Could you check a few things on this model? Use its own coordinates, in mm. A direction names the side the tool comes from. Round coordinates to 2 decimals unless told otherwise and drop trailing zeros. Write each loop counter-clockwise with the first axis right and the second up, starting at its lowest first coordinate (ties: lowest second). Pieces come first, ordered by that corner, then holes. Notation, with made-up numbers: (17.5, -0.5) - (43.5, -0.5) arc R15 ccw to (43.5, 14.5) - close; hole circle Ø11 at (34.25, 26). An arc over 180 degrees is marked (long way). Put each result on its own line as item: value.
Autodesk Fusion 360 part; units mm, degrees
sketch "Esquisse1" plane through (0, 0, 0) normal (0, 0, 1) x (1, 0, 0)
  line L0 (15.7988, 249.7948) -> (43.7076, 249.7948) construction
  line L1 (15.7988, 262.2639) -> (10.7166, 262.2639)
  line L2 (10.7166, 262.2639) -> (10.7166, 237.5139)
  line L3 (10.7166, 237.5139) -> (15.7988, 237.4198)
  line L4 (15.7988, 274.8948) -> (15.7988, 262.2639)
  line L5 (15.7988, 237.4198) -> (15.7988, 224.6948)
  line L6 (110.3988, 274.8948) -> (110.3988, 280.2948)
  line L7 (110.3988, 280.2948) -> (60.5988, 280.2948)
  line L8 (60.5988, 280.2948) -> (60.5988, 274.8948)
  line L9 (15.7988, 274.8948) -> (60.5988, 274.8948)
  line L10 (110.3988, 274.8948) -> (155.1988, 274.8948)
  line L11 (110.3988, 224.6948) -> (110.3988, 219.2948)
  line L12 (110.3988, 219.2948) -> (60.5988, 219.2948)
  line L13 (60.5988, 219.2948) -> (60.5988, 224.6948)
  line L14 (155.1988, 224.6948) -> (110.3988, 224.6948)
  line L15 (60.5988, 224.6948) -> (15.7988, 224.6948)
  line L16 (85.4988, 283.8421) -> (85.4988, 207.6137) construction
  line L17 (155.1988, 262.2639) -> (160.281, 262.2639)
  line L18 (160.281, 262.2639) -> (160.281, 237.5139)
  line L19 (160.281, 237.5139) -> (155.1988, 237.4198)
  line L20 (155.1988, 274.8948) -> (155.1988, 262.2639)
  line L21 (155.1988, 237.4198) -> (155.1988, 224.6948)
  circle A0 centre (13.4166, 249.7948) radius 1.6
  circle A1 centre (157.581, 249.7948) radius 1.6
  line L22 (33.7988, 274.8948) -> (37.1988, 274.8948)
  line L23 (37.1988, 274.8948) -> (37.1988, 268.8948)
  line L24 (33.7988, 268.8948) -> (33.7988, 274.8948)
  line L25 (35.4988, 277) -> (35.4988, 258) construction
  line L26 (32.7988, 268.8948) -> (32.7988, 266.1948)
  line L27 (38.1988, 266.1948) -> (38.1988, 268.8948)
  line L28 (37.1988, 266.1948) -> (37.1988, 264.6948)
  line L29 (36.6988, 264.1948) -> (34.2988, 264.1948)
  line L30 (33.7988, 264.6948) -> (33.7988, 266.1948)
  arc A2 (33.7988, 264.6948) -> (34.2988, 264.1948) centre (34.2988, 264.6948) ccw
  arc A3 (36.6988, 264.1948) -> (37.1988, 264.6948) centre (36.6988, 264.6948) ccw
  line L31 (32.7988, 266.1948) -> (33.7988, 266.1948)
  line L32 (37.1988, 266.1948) -> (38.1988, 266.1948)
  line L33 (38.1988, 268.8948) -> (37.1988, 268.8948)
  line L34 (33.7988, 268.8948) -> (32.7988, 268.8948)
  line L35 (33.7988, 234.8948) -> (33.7988, 233.3948)
  line L36 (37.1988, 233.3948) -> (38.1988, 233.3948)
  line L37 (38.1988, 233.3948) -> (38.1988, 230.6948)
  arc A4 (34.2988, 235.3948) -> (33.7988, 234.8948) centre (34.2988, 234.8948) ccw
  line L38 (32.7988, 230.6948) -> (32.7988, 233.3948)
  arc A5 (37.1988, 234.8948) -> (36.6988, 235.3948) centre (36.6988, 234.8948) ccw
  line L39 (36.6988, 235.3948) -> (34.2988, 235.3948)
  line L40 (37.1988, 233.3948) -> (37.1988, 234.8948)
  line L41 (32.7988, 233.3948) -> (33.7988, 233.3948)
  line L42 (33.7988, 230.6948) -> (32.7988, 230.6948)
  line L43 (38.1988, 230.6948) -> (37.1988, 230.6948)
  line L44 (33.7988, 230.6948) -> (33.7988, 224.6948)
  line L45 (37.1988, 224.6948) -> (37.1988, 230.6948)
  line L46 (138.1988, 268.8948) -> (138.1988, 266.1948)
  line L47 (137.1988, 230.6948) -> (138.1988, 230.6948)
  line L48 (133.7988, 233.3948) -> (133.7988, 234.8948)
  line L49 (132.7988, 268.8948) -> (133.7988, 268.8948)
  line L50 (138.1988, 233.3948) -> (137.1988, 233.3948)
  line L51 (132.7988, 266.1948) -> (132.7988, 268.8948)
  line L52 (133.7988, 266.1948) -> (133.7988, 264.6948)
  line L53 (133.7988, 266.1948) -> (132.7988, 266.1948)
  line L54 (132.7988, 233.3948) -> (132.7988, 230.6948)
  line L55 (137.1988, 268.8948) -> (138.1988, 268.8948)
  line L56 (137.1988, 234.8948) -> (137.1988, 233.3948)
  line L57 (138.1988, 230.6948) -> (138.1988, 233.3948)
  line L58 (134.2988, 264.1948) -> (136.6988, 264.1948)
  arc A6 (134.2988, 235.3948) -> (133.7988, 234.8948) centre (134.2988, 234.8948) ccw
  arc A7 (137.1988, 234.8948) -> (136.6988, 235.3948) centre (136.6988, 234.8948) ccw
  line L59 (132.7988, 230.6948) -> (133.7988, 230.6948)
  line L60 (138.1988, 266.1948) -> (137.1988, 266.1948)
  line L61 (137.1988, 264.6948) -> (137.1988, 266.1948)
  arc A8 (136.6988, 264.1948) -> (137.1988, 264.6948) centre (136.6988, 264.6948) ccw
  line L62 (134.2988, 235.3948) -> (136.6988, 235.3948)
  arc A9 (133.7988, 264.6948) -> (134.2988, 264.1948) centre (134.2988, 264.6948) ccw
  line L63 (133.7988, 233.3948) -> (132.7988, 233.3948)
  line L64 (137.1988, 230.6948) -> (137.1988, 224.6948)
  line L65 (133.7988, 224.6948) -> (133.7988, 230.6948)
  line L66 (137.1988, 268.8948) -> (137.1988, 274.8948)
  line L67 (133.7988, 274.8948) -> (133.7988, 268.8948)
  point P0 (155.1988, 249.7948)
  point P1 (33.7988, 264.1948)
  point P2 (33.7988, 235.3948)
  point P3 (127.2901, 249.7948)
  point P4 (137.1988, 235.3948)
  point P5 (135.4988, 258)
  point P6 (137.1988, 264.1948)
  dimension "d99" = 139.4
  dimension "d100" = 49.8
  dimension "d101" = 44.8
  dimension "d102" = 5.4
  dimension "d103" = 69.7
  dimension "d104" = 24.75
  dimension "d105" = 50.2
  dimension "d106" = 12.725
  dimension "d107" = 3.2
  dimension "d109" = 2.7
  dimension "d110" = 6
  dimension "d111" = 3.4
  dimension "d113" = 1.7
  dimension "d114" = 5.4
  dimension "d115" = 2.7
  dimension "d116" = 2.7
  dimension "d117" = 3.4
  dimension "d118" = 1.7
  dimension "d119" = 2
  dimension "d120" = 0.5
  dimension "d121" = 25.1
extrude "Extrusion1" add sketch "Esquisse1" along normal blind 5 contours L1 L2 L3 L4 L5 L6 L7 L8 L9 L10 L11 L12 L13 L14 L15 L17 L18 L19 L20 L21 L23 L24 L26 L27 L28 L29 L30 A2 A3 L31 L32 L33 L34 L35 L36 L37 A4 L38 A5 L39 L40 L41 L42 L43 L44 L45 L46 L47 L48 L49 L50 L51 L52 L53 L54 L55 L56 L57 L58 A6 A7 L59 L60 L61 A8 L62 A9 L63 L64 L65 L66 L67
equation "d84 = 5.3 mm + 0.1 mm"
equation "d87 = 36 mm - 0.2 mm"
equation "d88 = 36 mm + 0.1 mm"
equation "d101 = ( d99 - d100 ) / 2"
equation "d103 = d99 / 2"
equation "d106 = ( d105 - d104 ) / 2"
equation "d109 = d102 / 2"
equation "d113 = d111 / 2"
equation "d116 = d114 / 2"
equation "d117 = d111"
equation "d118 = d117 / 2"
(1) Imagine slicing it at A-A, the plane y = 229. List the corners of the cut face in (x, z) for me.
Values found:
outline: (15.8, 0) - (33.8, 0) - (33.8, 5) - (15.8, 5) - close; (37.2, 0) - (133.8, 0) - (133.8, 5) - (37.2, 5) - close; (137.2, 0) - (155.2, 0) - (155.2, 5) - (137.2, 5) - close
(2) Please list where these lines run through material, in increasing order: probe 1 along X at (y, z) = (269, 4.8); probe 2 along Y at (x, z) = (38, 4.4); probe 3 along Y at (x, z) = (123, 1.5). Write a range as from..to.
Values found:
probe 1: x = 15.8..33.8, 37.2..133.8, 137.2..155.2
probe 2: y = 224.69..230.69, 233.39..266.19, 268.89..274.89
probe 3: y = 224.69..274.89
(3) Imagine slicing it at C-C, the plane z = 1.6. Give the number of separate pieces and of enclosed holes in the cut face, then the cut area to 4 significant figures.
Values found:
separate pieces: 1
enclosed holes: 2
area: 7,605 mm^2
(4) I'm going to push flat-ended pins straight in: pin 1 (2.5 mm diameter, centred on x = 13.42, y = 249.79, fed in from +Z); pin 2 (0.8 mm diameter, centred on x = 137.5, z = 3, fed in from -Y); pin 3 (1.5 mm diameter, centred on y = 228, z = 2, fed in from +X); pin 4 (0.7 mm diameter, centred on x = 35, z = 3.5, fed in from -Y). Where does each tip first touch, or does it pass through?
Values found:
pin 1: passes through
pin 2: stops at y = 224.69
pin 3: stops at x = 155.2
pin 4: stops at y = 235.39
(5) Imagine slicing it at B-B, the plane x = 127.5. List the corners of the cut face in (y, z) for me, then the cut area to 3 significant figures.
Values found:
outline: (224.69, 0) - (274.89, 0) - (274.89, 5) - (224.69, 5) - close
area: 251 mm^2
(6) For faces 5 (the face through (122, 274.895, 2)), 6 (the face through (25, 224.695, 2)), 7 (the face through (146, 224.695, 2)), 8 (the face through (132.799, 232, 2)), which set-ups out of +Z, -Z, +X, -X, +Y, -Y let a thin tool reach every point of the face, with its end or its side?
Values found:
face 5: +Z, -Z, +X, +Y
face 6: +Z, -Z, -X, -Y
face 7: +Z, -Z, +X, -Y
face 8: +Z, -Z
(7) If we mould it in two halves opening along X, with no side actions, what happens to faces 1 (the face through (110.399, 278, 2)), 2 (the face through (133.799, 228, 2)), 3 (the face through (49, 224.695, 2)), 4 (the face through (60.599, 278, 2))? For each: pulls with the +X half, pulls with the -X half, needs draft (parallel to the pull), parting line crosses it, or undercut.
Values found:
face 1: pulls with the +X half
face 2: undercut
face 3: needs draft
face 4: pulls with the -X half
